Verification items for this drawing (mm, ordinates from the low corner). Round coordinates to 2 decimals unless told otherwise and drop trailing zeros. Order: outer loops, then holes, each group sorted by start corner. A loop starts at its lowest first (then second) coordinate and runs counter-clockwise, first axis right, second up. Notation, with made-up numbers: (31.5, 40) -> (49.5, 40) arc R23 cw to (49.5, 57) -> close; hole circle Ø10 at (64, 21). An arc over 180 degrees is marked (long way). Put each result on its own line as item: value.
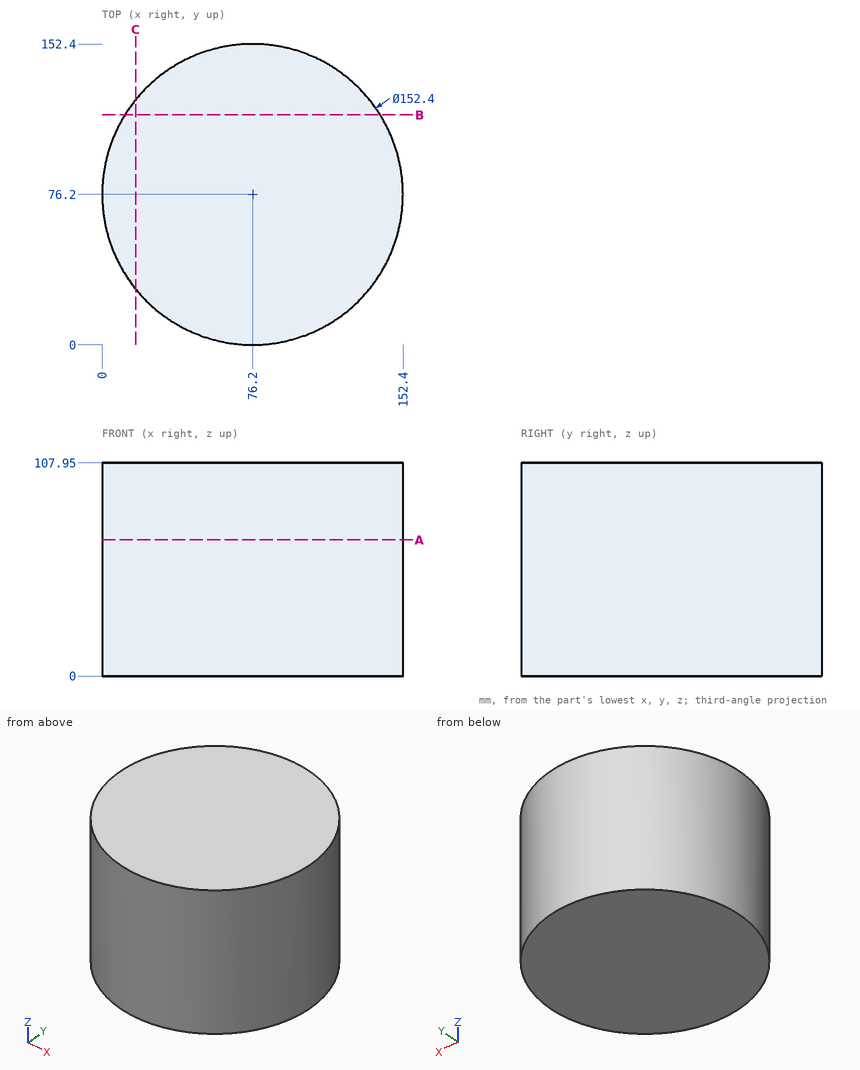
Item 1: Gauge pin test, flat ends, axial feed: pin 1 Ø12 at (x, z) = (46, 95.5) entering from +Y; pin 2 Ø10 at (y, z) = (33, 76.5) entering from -X; pin 3 Ø5 at (x, z) = (79.5, 74) entering from +Y. Record the tip position at first contact, or that the pin passes through.
Check sheet entries:
pin 1: stops at y = 148.46
pin 2: stops at x = 10.27
pin 3: stops at y = 152.4
Item 2: Section check A-A on z = 69. Record the boundary of the cut face in (x, y), then the cut area to 3 significant figures.
Check sheet entries:
outline: circle Ø152.4 at (76.2, 76.2)
area: 18,200 mm^2
Item 3: Material ranges on L1, parallel to Y at x = 50, z = 23; L2, parallel to Y at x = 32, z = 65; L3, parallel to X at y = 139.5, z = 10, recorded low to high. Write a range as [from, to].
Check sheet entries:
L1: y = [4.65, 147.75]
L2: y = [14.13, 138.27]
L3: x = [33.78, 118.62]
Item 4: Section check C-C on x = 17. Record the boundary of the cut face in (y, z), then the cut area to 3 significant figures.
Check sheet entries:
outline: (28.22, 0) -> (124.18, 0) -> (124.18, 107.95) -> (28.22, 107.95) -> close
area: 10,400 mm^2
Item 5: Section check B-B on y = 116.5. Record the boundary of the cut face in (x, z), then the cut area to 3 significant figures.
Check sheet entries:
outline: (11.53, 0) -> (140.87, 0) -> (140.87, 107.95) -> (11.53, 107.95) -> close
area: 14,000 mm^2
